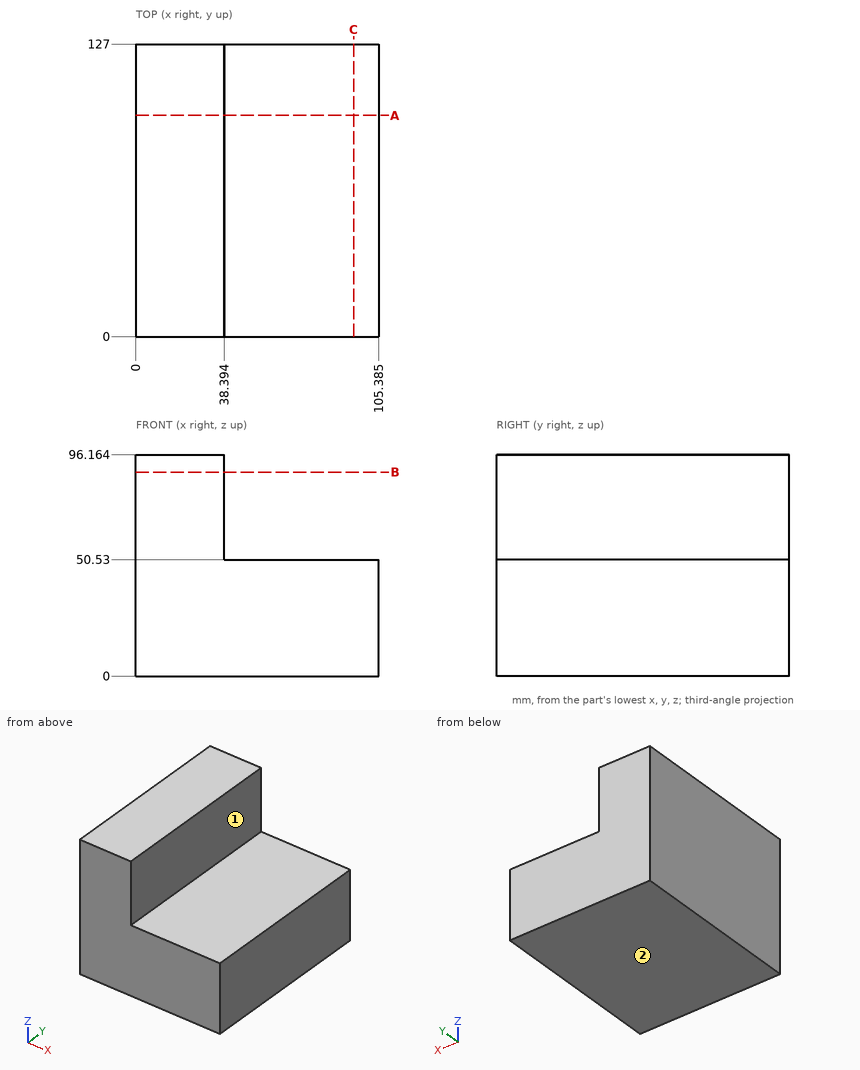
Print and shaded views of the part. All mm, measured from the part's lowest x, y and z. A direction names the side the tool comes from. Give positions to 0.01 mm unless a question says otherwise; leave off trailing zeros. Loops run counter-clockwise (first coordinate to the right, second up) from the corner with the lowest first, then second, coordinate; pieces in that order, holes last.
1) Saw through at C-C (x = 94.5). Write the cut outline in (y, z), plus the area to 3 significant figures.
2) Saw through at A-A (y = 96). Write the cut outline in (x, z) (1 decimal).
3) Flat gauge pins, fed straight in: pin 1 Ø3 at (y, z) = (102.5, 52) entering from +X (1 decimal); pin 2 Ø1 at (x, y) = (65, 22) entering from +Z. Where does each tip first touch, or does it go through?
4) Tool access for the marked faces 1 and 2: list every direction of +Z, -Z, +X, -X, +Y, -Y with a clear straight run to the whole face (end or side of a thin tool).
5) Saw through at B-B (z = 88.5). Write the cut outline in (x, y) (1 decimal), plus the area to 3 significant figures.
6) Wall check: line 1 (X direction, y = 22, z = 78) (1 decimal); line 2 (Z direction, x = 48.5, y = 92.5). Give the ranges that are in metal, low to high.
Answer block:
1. outline: (0, 0) - (127, 0) - (127, 50.53) - (0, 50.53) - close
1. area: 6,420 mm2
2. outline: (0, 0) - (105.4, 0) - (105.4, 50.5) - (38.4, 50.5) - (38.4, 96.2) - (0, 96.2) - close
3. pin 1: stops at x = 105.4
3. pin 2: stops at z = 50.53
4. face 1: +Z, +X, +Y, -Y
4. face 2: -Z, +X, -X, +Y, -Y
5. outline: (0, 0) - (38.4, 0) - (38.4, 127) - (0, 127) - close
5. area: 4,880 mm2
6. line 1: x = 0 to 38.4
6. line 2: z = 0 to 50.53
